Check sheet for the drawn part. Datum: minimum x, y, z corner. Units: mm. Round coordinates to 2 decimals unless told otherwise and drop trailing zeros. Loops run counter-clockwise (first coordinate to the right, second up) from the corner with the lowest first, then second, coordinate; pieces in that order, holes last. Notation, with made-up numbers: (57, 33.25) -> (116, 33.25) arc R13 cw to (116, 50.25) -> close; hole circle Ø1 at (51.5, 26). An arc over 180 degrees is marked (long way). Return JSON: item names as keys, results as strings.
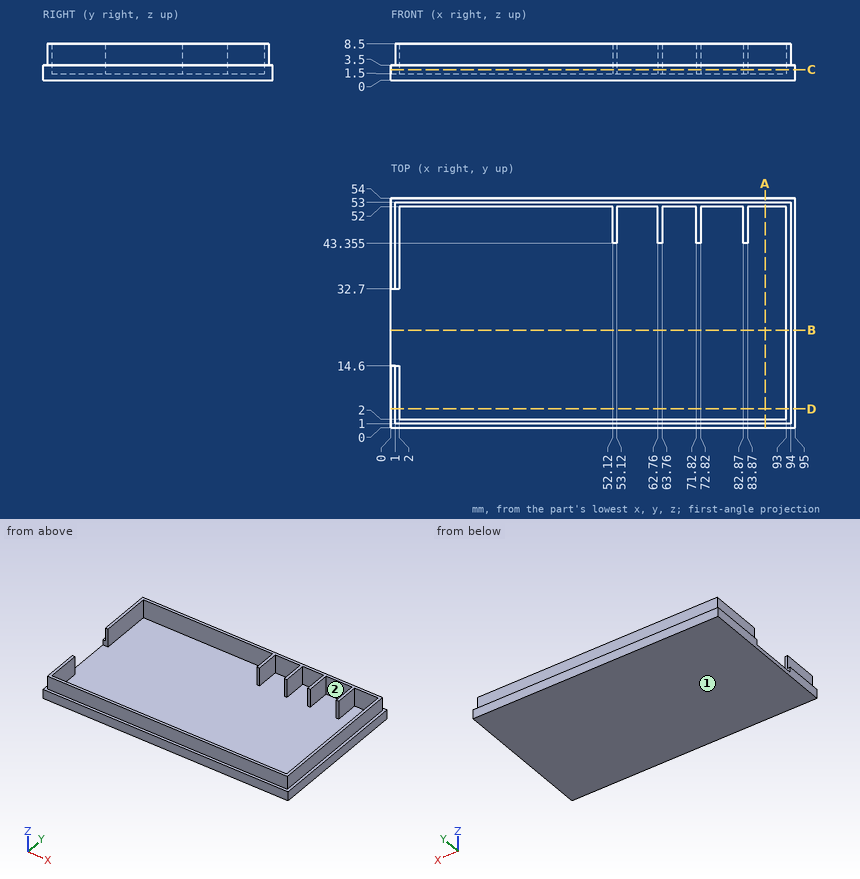
Q1. Section check D-D (y = 4.5). Record the boundary of the cut face in (x, z).
Results list:
{"outline": "(0, 0) -> (95, 0) -> (95, 3.5) -> (94, 3.5) -> (94, 8.5) -> (93, 8.5) -> (93, 1.5) -> (2, 1.5) -> (2, 8.5) -> (1, 8.5) -> (1, 3.5) -> (0, 3.5) -> close"}
Q2. Go/stop test with flat-tipped pins: pin 1 (3.5 mm diameter, centred on x = 58, z = 3.5, fed in from -Y); pin 2 (1.6 mm diameter, centred on x = 1, z = 5.5, fed in from -Y); pin 3 (1.5 mm diameter, centred on y = 29.5, z = 6.5, fed in from +X); pin 4 (1 mm diameter, centred on x = 68, z = 4.5, fed in from +Y). Record where each tip stops, or that it passes through.
Results list:
{"pin 1": "y = 0", "pin 2": "y = 1", "pin 3": "x = 94", "pin 4": "y = 53"}
Q3. Material ranges on line 1 (Y direction, x = 61.5, z = 4.75); line 2 (Y direction, x = 33, z = 3.25); line 3 (X direction, y = 47.5, z = 5.25), recorded low to high.
Results list:
{"line 1": "1 to 2, 52 to 53", "line 2": "0 to 2, 52 to 54", "line 3": "1 to 2, 52.12 to 53.12, 62.76 to 63.76, 71.82 to 72.82, 82.87 to 83.87, 93 to 94"}
Q4. Section check A-A (x = 88). Record the boundary of the cut face in (y, z), then the cut area to 3 significant figures.
Results list:
{"outline": "(0, 0) -> (54, 0) -> (54, 3.5) -> (53, 3.5) -> (53, 8.5) -> (52, 8.5) -> (52, 1.5) -> (2, 1.5) -> (2, 8.5) -> (1, 8.5) -> (1, 3.5) -> (0, 3.5) -> close", "area": "99.0 mm^2"}
Q5. Section check B-B (y = 23). Record the boundary of the cut face in (x, z).
Results list:
{"outline": "(0, 0) -> (95, 0) -> (95, 3.5) -> (94, 3.5) -> (94, 8.5) -> (93, 8.5) -> (93, 1.5) -> (0, 1.5) -> close"}
Q6. Section check C-C (z = 2.5). Record the boundary of the cut face in (x, y) (1 decimal).
Results list:
{"outline": "(0, 0) -> (95, 0) -> (95, 54) -> (0, 54) -> (0, 32.7) -> (2, 32.7) -> (2, 52) -> (52.1, 52) -> (52.1, 43.4) -> (53.1, 43.4) -> (53.1, 52) -> (62.8, 52) -> (62.8, 43.4) -> (63.8, 43.4) -> (63.8, 52) -> (71.8, 52) -> (71.8, 43.4) -> (72.8, 43.4) -> (72.8, 52) -> (82.9, 52) -> (82.9, 43.4) -> (83.9, 43.4) -> (83.9, 52) -> (93, 52) -> (93, 2) -> (2, 2) -> (2, 14.6) -> (0, 14.6) -> close"}
Q7. Draft check along X on the marked faces 1 and 2. Enter one of: released by +X, released by -X, zero draft, split by the parting line, or undercut.
Results list:
{"face 1": "zero draft", "face 2": "undercut"}
